```python
from build123d import *

# Parameters (mm, degrees)
SWEEP1_PROFILE_R    = 11
SKETCH34_R          = 11
BOSS_EXTRUDE1_DEPTH = 7.5
SKETCH41_R          = 11.5
BOSS_EXTRUDE2_DEPTH = 2
SKETCH42_R          = 10
BOSS_EXTRUDE3_DEPTH = 500
SKETCH43_R          = 11.5
BOSS_EXTRUDE4_DEPTH = 7.5
SKETCH129_R         = 7.5
BOSS_EXTRUDE5_DEPTH = 3


with BuildPart() as part:
    # Sweep1: sweep along a path in Sketch1
    with BuildLine(Plane(origin=(0, 0, 0), x_dir=(1, 0, 0), z_dir=(0, 1, 0))) as sweep1_path:
        Line((-112.299146126, 73.980831747), (-112.299146126, 84.480831747))
        ThreePointArc((-112.299146126, 84.480831747), (-108.93087411, 92.612559731), (-100.799146126, 95.980831747))
        Line((-100.799146126, 95.980831747), (-83.999146126, 95.980831747))
    # Sweep1 profile (on start of the path) → Sweep1 (sweep)
    with BuildSketch(Plane(origin=(-112.299146126, 0, -73.980831747), x_dir=(-1, 0, 0), z_dir=(0, 0, -1))):
        Circle(SWEEP1_PROFILE_R)
    sweep(path=sweep1_path.line)

    # Sketch34 → Boss-Extrude1 (add)
    with BuildSketch(Plane.XY.offset(-73.980831747)):
        with Locations((-112.299146126, 0)):
            Circle(SKETCH34_R)
    extrude(amount=BOSS_EXTRUDE1_DEPTH)

    # Sketch41 → Boss-Extrude2 (add)
    with BuildSketch(Plane(origin=(-83.999146126, 0, 0), x_dir=(0, 0, -1), z_dir=(1, 0, 0))):
        with Locations((95.980831747, 0)):
            Circle(SKETCH41_R)
    extrude(amount=BOSS_EXTRUDE2_DEPTH)

    # Sketch42 → Boss-Extrude3 (add)
    with BuildSketch(Plane.XY.offset(-66.480831747)):
        with Locations((-112.299146126, 0)):
            Circle(SKETCH42_R)
    extrude(amount=BOSS_EXTRUDE3_DEPTH)

    # Sketch43 → Boss-Extrude4 (add)
    with BuildSketch(Plane.XY.offset(433.519168253)):
        with Locations((-112.299146126, 0)):
            Circle(SKETCH43_R)
    extrude(amount=BOSS_EXTRUDE4_DEPTH)

    # Sketch129 → Boss-Extrude5 (add)
    with BuildSketch(Plane(origin=(-81.999146126, 0, 0), x_dir=(0, 0, -1), z_dir=(1, 0, 0))):
        with Locations((95.980831747, 0)):
            Circle(SKETCH129_R)
    extrude(amount=BOSS_EXTRUDE5_DEPTH)


solid = part.part
```
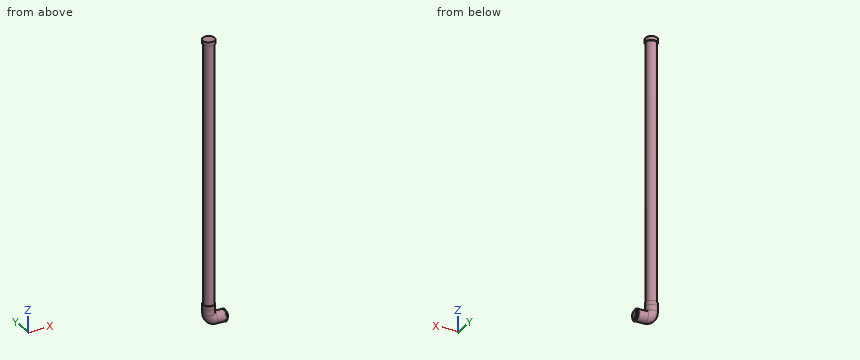
Geometry: final body of the model. Coordinates: model frame, mm. Give positions to 0.01 mm unless a question says otherwise; leave off trailing zeros. Loops run counter-clockwise (first coordinate to the right, second up) from the corner with the lowest first, then second, coordinate; pieces in that order, holes last. Notation, with made-up numbers: (76, 63) -> (104, 63) arc R31 cw to (104, 101) -> close; hole circle Ø10 at (-27, 4). An arc over 180 degrees is marked (long way). Return JSON: item names as keys, results as strings.
Item 1: Section C-C, the plane x = -89.5. Output: boundary loops of the cut face in (y, z).
Filled in:
{"outline": "circle Ø22 at (0, -95.98)"}
Item 2: Pin query (flat end, axial travel): P1, Ø6, axis at y = 1.5, z = 270, coming from the -X side; P2, Ø10, axis at y = 9, z = 42, coming from the -X side; P3, Ø2, axis at x = -100.5, y = -4, coming from the -Z side. Return the tip coordinate at first contact, or that it passes through.
Filled in:
{"P1": "x = -122.3", "P2": "x = -121.46", "P3": "z = -106.56"}
Item 3: Line query: line 1 (Y direction, x = -119, z = 135); line 2 (Y direction, x = -111, z = 223.5); line 3 (Z direction, x = -112.5, y = -2). Output: solid intervals per line, ascending.
Filled in:
{"line 1": "-7.42 to 7.42", "line 2": "-9.92 to 9.92", "line 3": "-103.48 to 441.02"}
Item 4: Section A-A, the plane y = 0. Output: boundary loops of the cut face in (x, z), plus the area to 3 significant figures.
Filled in:
{"outline": "(-123.8, 433.52) -> (-122.3, 433.52) -> (-122.3, -66.48) -> (-123.3, -66.48) -> (-123.3, -84.48) arc R22.5 ccw to (-100.8, -106.98) -> (-84, -106.98) -> (-84, -107.48) -> (-82, -107.48) -> (-82, -103.48) -> (-79, -103.48) -> (-79, -88.48) -> (-82, -88.48) -> (-82, -84.48) -> (-84, -84.48) -> (-84, -84.98) -> (-100.8, -84.98) arc R0.5 cw to (-101.3, -84.48) -> (-101.3, -66.48) -> (-102.3, -66.48) -> (-102.3, 433.52) -> (-100.8, 433.52) -> (-100.8, 441.02) -> (-123.8, 441.02) -> close", "area": "11,400 mm^2"}
Item 5: Section B-B, the plane z = 127.5. Output: boundary loops of the cut face in (x, y).
Filled in:
{"outline": "circle Ø20 at (-112.3, 0)"}
